Input: dimensioned drawing with shaded views. Units: mm. Origin: part minimum x, y, z. A direction names the side the tool comes from. Round coordinates to 2 decimals unless told otherwise and drop trailing zeros. Order: outer loops, then holes, each group sorted by start corner. A loop starts at its lowest first (then second) coordinate and runs counter-clockwise, first axis right, second up. Notation, with made-up numbers: (-37.75, 42) -> (-32.75, 42) arc R24 ccw to (-32.75, 64) -> close; hole circle Ø3 at (89, 37). An arc over 180 degrees is marked (long way). Use a Markdown table: item, result. Add a question column.
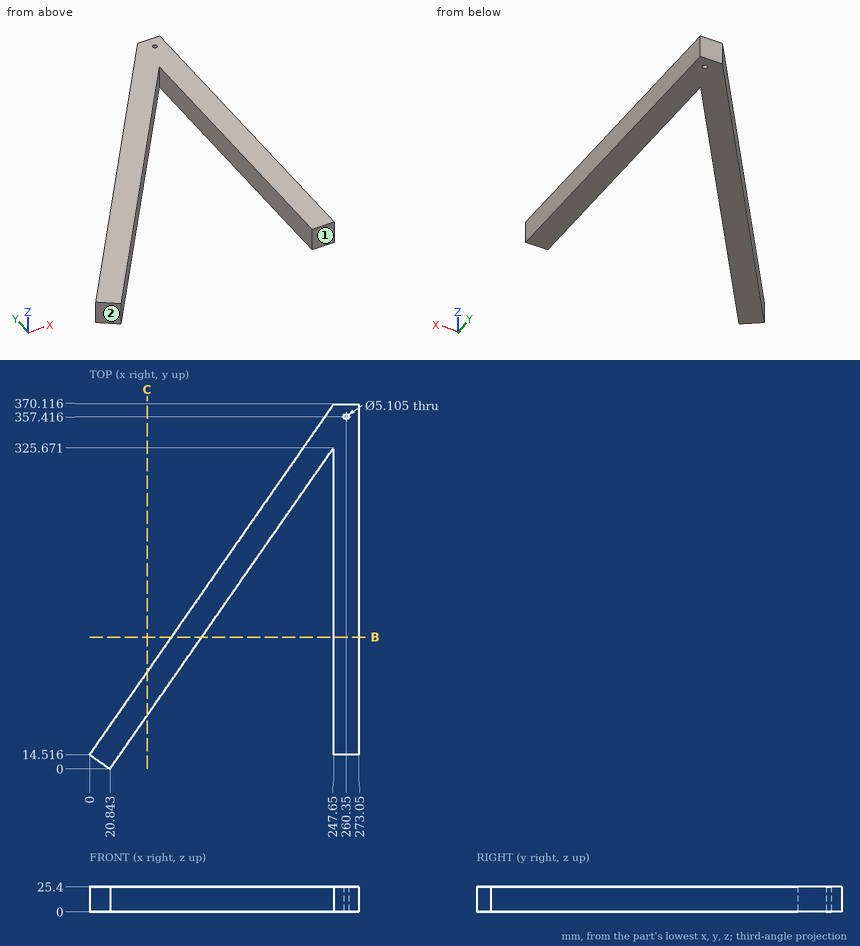
1) Section B-B on y = 133.5. Output: boundary loops of the cut face in (x, z).
2) First-contact query: pin 1 Ø8 at (x, z) = (92.5, 18) entering from -Y; pin 2 Ø7.5 at (y, z) = (105.5, 11) entering from -X; pin 3 Ø4 at (x, z) = (80, 12.5) entering from +Y; pin 4 Ø1.5 at (x, y) = (131.5, 193) entering from -Z. Flat tips, straight axial feed; report the tip coordinate or a pass-through.
3) Section C-C on x = 58.5. Output: boundary loops of the cut face in (y, z), then the cut area to 3 significant figures.
4) Line query: probe 1 along X at (y, z) = (20, 8); probe 2 along X at (y, z) = (272, 19); probe 3 along Y at (x, z) = (183.5, 6.5) (1 decimal). Output: solid intervals per line, ascending. Write a range as from..to.
5) Reachability of the marked faces 1 and 2 from +Z, -Z, +X, -X, +Y, -Y: full face, straight path, thin tool, end or side. Return the list, or none.
Conclusion:
| question | item | result |
|---|---|---|
| 1 | outline | (82.86, 0) -> (113.82, 0) -> (113.82, 25.4) -> (82.86, 25.4) -> close; (247.65, 0) -> (273.05, 0) -> (273.05, 25.4) -> (247.65, 25.4) -> close |
| 2 | pin 1 | stops at y = 97.15 |
| 2 | pin 2 | stops at x = 60.75 |
| 2 | pin 3 | stops at y = 132.26 |
| 2 | pin 4 | stops at z = 0 |
| 3 | outline | (54.07, 0) -> (98.52, 0) -> (98.52, 25.4) -> (54.07, 25.4) -> close |
| 3 | area | 1,130 mm^2 |
| 4 | probe 1 | x = 3.82..34.77, 247.65..273.05 |
| 4 | probe 2 | x = 179.32..210.27, 247.65..273.05 |
| 4 | probe 3 | y = 233.6..278 |
| 5 | face 1 | +Z, -Z, +X, -Y |
| 5 | face 2 | +Z, -Z, -X, -Y |
